The model under review builds one solid part; all positions refer to its coordinate system, in mm. A direction names the side the tool comes from. Coordinates: 2 decimals unless noted, no trailing zeros. Order: outer loops, then holes, each group sorted by start corner. A loop starts at its lowest first (then second) coordinate and runs counter-clockwise, first axis right, second up. Notation, with made-up numbers: M 88.25,88 L 97.25,88 A11 cw 97.25,109 Z; hole C 15.5,-9.75 d8. An arc over 180 degrees is marked long. Write each question's results on one line, items separated by ' | '.
from build123d import *

# Parameters (mm, degrees)
F0_W     = 37.809022
F0_H     = 30.170836
F1_DEPTH = 25.4
F4_W     = 43.719644
F4_H     = 120.03813
F5_DEPTH = 2.54


with BuildPart() as f1:
    # F0 (on Top) → F1 (new body)
    with BuildSketch(Plane.XY):
        Rectangle(F0_W, F0_H)
    extrude(amount=F1_DEPTH)


with BuildPart() as f5:
    # F4 (on face) → F5 (new body)
    with BuildSketch(Plane(origin=(14.130645, 0, -14.130645), x_dir=(0.707107, 0, 0.707107), z_dir=(-0.707107, 0, 0.707107))):
        with Locations((10.187182, -33.240173)):
            Rectangle(F4_W, F4_H)
    extrude(amount=F5_DEPTH)


with BuildPart() as f5_1:
    # F6: moved
    add(f5.part.moved(Location((-19.5326, 0, 0))))


with BuildPart() as f1_1:
    add(f1.part)

    # F7: cut F5
    add(f5_1.part, mode=Mode.SUBTRACT)


solid = f1_1.part
1) For pin 1 (1.5 mm diameter, centred on x = -8.5, y = -9, fed in from -Z), flat-tipped, find the tip position at first contact; note if it passes through.
Solutions:
pin 1: z = 0
2) Take a section at C-C on x = 16.5. State the section outline as (y, z) points.
Solutions:
outline: M -15.09,0 L 15.09,0 L 15.09,7.77 L -15.09,7.77 Z; M -15.09,9.29 L 15.09,9.29 L 15.09,25.4 L -15.09,25.4 Z
3) To check wall thickness, follow line 1 along Z through (x, y) = (14, 3); line 2 along X through (y, z) = (-11, 10.25); line 3 along X through (y, z) = (9, 4.75). State the ranges of each line that lie inside material, in increasing order.
Solutions:
line 1: 0 to 5.27, 8.86 to 25.4 | line 2: -18.9 to 15.39, 15.54 to 18.9 | line 3: -18.9 to 9.89, 13.48 to 18.9
4) The part is to be moulded in two halves that separate along Z. For faces 1 (the flat face through (0, 0, 25.4)), 2 (the flat face through (0, -15.085, 13)), 3 (the flat face through (16.37, -0.21, 9.42)), 4 (the flat face through (-7, 0, 0)), say which applies: pulls with the +Z half, pulls with the -Z half, needs draft (parallel to the pull), parting line crosses it, or undercut.
Solutions:
face 1: pulls with the +Z half | face 2: needs draft | face 3: undercut | face 4: pulls with the -Z half
5) For faces 5 (the flat face through (10.227, 0.211, 5.091)), 6 (the flat face through (0, 15.085, 13)), list the 3-axis set-ups (+Z, -Z, +X, -X, +Y, -Y) from which the entire face can be reached by the end or side of a thin tool; tool diameter is ignored.
Solutions:
face 5: +Y, -Y | face 6: +Z, -Z, +X, -X, +Y
6) Take a section at D-D on x = 8. State the section outline as (y, z) points, plus the area to 3 significant figures.
Solutions:
outline: M -15.09,2.86 L 15.09,2.86 L 15.09,25.4 L -15.09,25.4 Z | area: 680 mm2
7) Take a section at B-B on y = 5. State the section outline as (x, z) points.
Solutions:
outline: M -18.9,0 L 5.14,0 L 15.46,10.33 L 17.26,8.53 L 8.73,0 L 18.9,0 L 18.9,25.4 L -18.9,25.4 Z
8) Take a section at A-A on z = 9.5. State the section outline as (x, y) points.
Solutions:
outline: M -18.9,-15.09 L 14.64,-15.09 L 14.64,15.09 L -18.9,15.09 Z; M 16.29,-15.09 L 18.9,-15.09 L 18.9,15.09 L 16.29,15.09 Z
